Here's how the part is built. I have some questions about the finished solid (model axes, mm). A direction names the side the tool comes from. Round coordinates to 2 decimals unless told otherwise and drop trailing zeros. Write each loop counter-clockwise with the first axis right and the second up, starting at its lowest first coordinate (ties: lowest second). Pieces come first, ordered by that corner, then holes. Notation, with made-up numbers: M 81,-39 L 98,-39 A14 cw 98,-12 Z; hole C 41,-12 d2. An arc over 180 degrees is marked long. Use a Markdown table: item, result. Add a question column.
```python
from build123d import *

# Parameters (mm, degrees)
F0_R      = 11
F1_DEPTH  = 4
F2_R      = 3.5
F3_DEPTH  = 4
F4_COUNT  = 6
F5_R      = 6
F6_DEPTH  = 4
F8_DEPTH  = 3.5
F9_R      = 1.55
F10_DEPTH = 8.001


with BuildPart() as f1:
    # F0 (on Top) → F1 (new body)
    with BuildSketch(Plane.XY):
        Circle(F0_R)
    extrude(amount=F1_DEPTH)

    # F4: F3 ×6 about axis
    f4_axis = Axis((0, 0, 4), (0, 0, 1))


with BuildPart() as f3:
    # F2 (on face) → F3 (new body, through all)
    with BuildSketch(Plane.XY.offset(4)):
        with Locations((0.2514506495, 10.9971256504)):
            Circle(F2_R)
    extrude(amount=-F3_DEPTH)


with BuildPart() as f1_1:
    add(f1.part)
    for i in range(1, F4_COUNT):
        add(f3.part.rotate(f4_axis, i * 360 / F4_COUNT), mode=Mode.SUBTRACT)

    # F4#seed: cut F3
    add(f3.part, mode=Mode.SUBTRACT)

    # F5 (on face) → F6 (join)
    with BuildSketch(Plane.XY.offset(4)):
        Circle(F5_R)
    extrude(amount=F6_DEPTH)

    # F7 (on face) → F8 (cut)
    with BuildSketch(Plane(origin=(0, 0, 0), x_dir=(1, 0, 0), z_dir=(0, 0, -1))):
        Polygon((1.6743157806, 2.9), (-1.6743157806, 2.9), (-3.3486315613, 0), (-1.6743157806, -2.9), (1.6743157806, -2.9), (3.3486315613, 0), align=None)
    extrude(amount=-F8_DEPTH, mode=Mode.SUBTRACT)

    # F9 (on face) → F10 (cut, through all)
    with BuildSketch(Plane.XY.offset(8)):
        Circle(F9_R)
    extrude(amount=-F10_DEPTH, mode=Mode.SUBTRACT)


solid = f1_1.part
```
Item 1: On a 3-axis mill with a long thin cutter (end or side, diameter ignored), from which of +Z, -Z, +X, -X, +Y, -Y can I reach the whole of each face in a straight line? I mean faces 5 (the face through (-6, 0, 6)), 6 (the face through (2.5, 1.47, 1.73)), 7 (the face through (6.444, -3.839, 2.028)). Say none if no direction works.
Item 2: For pin 1 Ø1.7 at (x, z) = (0.5, 2.5) entering from +Y; pin 2 Ø3 at (x, y) = (0, 0) entering from -Z; pin 3 Ø1 at (x, z) = (-0.5, 1.5) entering from -Y; pin 4 Ø4 at (x, z) = (-8, 1) entering from -Y, each with a flat end and sliding along its axis, tell me the tip position at first contact or that it passes through.
Item 3: Imagine slicing it at B-B on x = 0. List the corners of the cut face in (y, z) for me, plus the area to 3 significant figures.
Item 4: Imagine slicing it at D-D on y = 4.75. List the corners of the cut face in (x, z) for me.
Item 5: Imagine slicing it at A-A on z = 1. List the corners of the cut face in (x, y) for me, plus the area to 3 significant figures.
Item 6: Imagine slicing it at C-C on y = -9. List the corners of the cut face in (x, z) for me, plus the area to 3 significant figures.
Item 7: I need wall thicknesses on probe 1 along Y at (x, z) = (0, 6); probe 2 along Y at (x, z) = (-7, 3); probe 3 along Z at (x, y) = (3.5, -5.5). Which ranges of each line are inside material? Lowest first, please. Write a range as from..to.
Item 8: If we mould it in two halves opening along Y, with no side actions, what happens to faces 1 (the face through (-6.444, 3.839, 2.028)), 2 (the face through (0.715, -1.375, 5.781)), 3 (the face through (5.743, 9.382, 1.972)), 4 (the face through (1.25, -1.25, 8))? For each: +Y half, -Y half, draft (parallel to the pull), parting line (faces both ways), or undercut.
The answers:
| question | item | result |
|---|---|---|
| 1 | face 5 | +Z |
| 1 | face 6 | -Z |
| 1 | face 7 | +Z, -Z |
| 2 | pin 1 | y = 7.67 |
| 2 | pin 2 | through |
| 2 | pin 3 | y = -7.58 |
| 2 | pin 4 | y = -9.22 |
| 3 | outline | M -7.51,0 L -2.9,0 L -2.9,3.5 L -1.55,3.5 L -1.55,8 L -6,8 L -6,4 L -7.51,4 Z; M 1.55,3.5 L 2.9,3.5 L 2.9,0 L 7.51,0 L 7.51,4 L 6,4 L 6,8 L 1.55,8 Z |
| 3 | area | 73.8 mm² |
| 4 | outline | M -6.03,0 L 6.19,0 L 6.19,4 L 3.67,4 L 3.67,8 L -3.67,8 L -3.67,4 L -6.03,4 Z |
| 5 | outline | M -10.82,-1.98 A3.5 cw -7.5,-8.04 A11 ccw -3.69,-10.36 A3.5 cw 3.22,-10.52 A11 ccw 7.13,-8.38 A3.5 cw 10.72,-2.47 A11 ccw 10.82,1.98 A3.5 cw 7.5,8.04 A11 ccw 3.69,10.36 A3.5 cw -3.22,10.52 A11 ccw -7.13,8.38 A3.5 cw -10.72,2.47 A11 ccw Z; hole M -3.35,0 L -1.67,-2.9 L 1.67,-2.9 L 3.35,0 L 1.67,2.9 L -1.67,2.9 Z |
| 5 | area | 243 mm² |
| 6 | outline | M -6.32,0 L -3.13,0 L -3.13,4 L -6.32,4 Z; M 2.62,0 L 6.32,0 L 6.32,4 L 2.62,4 Z |
| 6 | area | 27.6 mm² |
| 7 | probe 1 | -6..-1.55, 1.55..6 |
| 7 | probe 2 | -8.49..-7.57, -2.99..3.17, 8.27..8.49 |
| 7 | probe 3 | 0..4 |
| 8 | face 1 | undercut |
| 8 | face 2 | undercut |
| 8 | face 3 | +Y half |
| 8 | face 4 | draft |
